Verification items for the finished model (mm, model axes). Coordinates: 2 decimals unless noted, no trailing zeros. Loops run counter-clockwise (first coordinate to the right, second up) from the corner with the lowest first, then second, coordinate; pieces in that order, holes last. Notation, with made-up numbers: (54.25, -23) - (81.25, -23) arc R8 cw to (81.25, -12) - close; hole circle Ø10 at (21, 78.5). An arc over 180 degrees is marked (long way). Answer as CSV lines item,"result". Start each with the question number.
1. Gauge pin test, flat ends, axial feed: P1, Ø12, axis at x = 40.5, y = -8, coming from the +Z side; P2, Ø1.5, axis at x = 68, z = 2.5, coming from the -Y side; P3, Ø1.5, axis at x = 51, z = 2, coming from the +Y side. Record the tip position at first contact, or that the pin passes through.
2. Cross-section at A-A (z = 1.9). State how many separate pieces and enclosed holes the cut face has, plus the area to 3 significant figures.
3. Material ranges on line 1 (Y direction, x = -18, z = 0.8); line 2 (Z direction, x = 44, y = 30.5); line 3 (Y direction, x = 68.5, z = 1.15), recorded low to high. Write a range as [from, to].
4. Cross-section at D-D (y = 29.5). Enter the section's corners in (x, z), plus the area to 3 significant figures.
5. Cross-section at B-B (x = 60.5). Enter the section's corners in (y, z), plus the area to 3 significant figures.
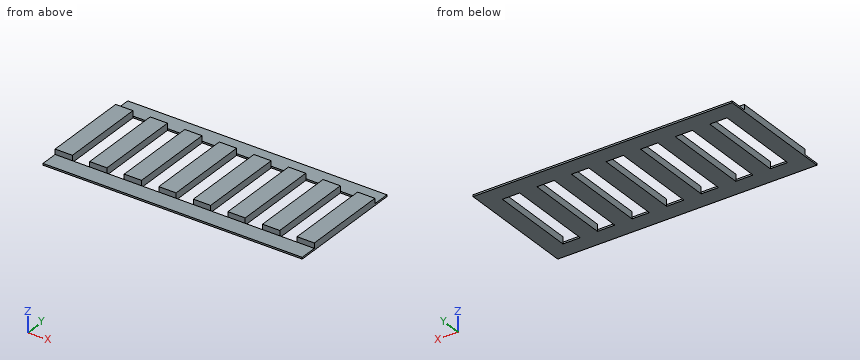
Autodesk Fusion 360 part; units mm, degrees
sketch "Sketch1" plane through (0, 0, 0) normal (0, 0, 1) x (1, 0, 0)
  line L0 (75, -35) -> (-75, -35)
  line L1 (-75, -35) -> (-75, 35)
  line L2 (-75, 35) -> (75, 35)
  line L3 (75, 35) -> (75, -35)
  line L4 (75, -35) -> (-75, 35) construction
  line L5 (-75, -35) -> (75, 35) construction
  line L6 (75, -25) -> (-75, -25)
  line L7 (-75, -25) -> (-75, 25)
  line L8 (-75, 25) -> (75, 25)
  line L9 (75, 25) -> (75, -25)
  line L10 (75, -25) -> (-75, 25) construction
  line L11 (-75, -25) -> (75, 25) construction
  line L12 (-75, 25) -> (-65, 25)
  line L13 (-65, 25) -> (-65, -25)
  line L14 (-65, -25) -> (-75, -25)
  line L15 (-75, -25) -> (-75, 25)
  line L16 (-55, 25) -> (-45, 25)
  line L17 (-45, 25) -> (-45, -25)
  line L18 (-45, -25) -> (-55, -25)
  line L19 (-55, -25) -> (-55, 25)
  line L20 (-35, 25) -> (-25, 25)
  line L21 (-25, 25) -> (-25, -25)
  line L22 (-25, -25) -> (-35, -25)
  line L23 (-35, -25) -> (-35, 25)
  line L24 (-15, 25) -> (-5, 25)
  line L25 (-5, 25) -> (-5, -25)
  line L26 (-5, -25) -> (-15, -25)
  line L27 (-15, -25) -> (-15, 25)
  line L28 (5, 25) -> (15, 25)
  line L29 (15, 25) -> (15, -25)
  line L30 (15, -25) -> (5, -25)
  line L31 (5, -25) -> (5, 25)
  line L32 (25, 25) -> (35, 25)
  line L33 (35, 25) -> (35, -25)
  line L34 (35, -25) -> (25, -25)
  line L35 (25, -25) -> (25, 25)
  line L36 (45, 25) -> (55, 25)
  line L37 (55, 25) -> (55, -25)
  line L38 (55, -25) -> (45, -25)
  line L39 (45, -25) -> (45, 25)
  line L40 (65, 25) -> (75, 25)
  line L41 (75, 25) -> (75, -25)
  line L42 (75, -25) -> (65, -25)
  line L43 (65, -25) -> (65, 25)
  dimension "d1" = 150
  dimension "d2" = 70
  dimension "d3" = 150
  dimension "d4" = 50
  dimension "d5" = 10
  dimension "d8" = 140
  dimension "d9" = 0
extrude "Extrude1" add sketch "Sketch1" along normal blind 4 contours L3 L6 L8 L9 L40 L41 L42 L43 | L1 L6 L7 L8 L12 L13 L14 L15 | L6 L8 L36 L37 L38 L39 | L6 L8 L16 L17 L18 L19 | L6 L8 L32 L33 L34 L35 | L6 L8 L20 L21 L22 L23 | L6 L8 L28 L29 L30 L31 | L6 L8 L24 L25 L26 L27 makes body 1 at (-31.6667, 8.3333, 0) makes body 2 at (-71.6667, 8.3333, 0) makes body 3 at (31.6667, -8.3333, 0) makes body 4 at (-51.6667, 8.3333, 0) makes body 5 at (68.3333, -8.3333, 0) makes body 6 at (11.6667, -8.3333, 0) makes body 7 at (51.6667, -8.3333, 0) makes body 8 at (-11.6667, 8.3333, 0)
extrude "Extrude2" add sketch "Sketch1" along normal blind 1 contours L0 L1 L3 L6 L14 L18 L22 L26 L30 L34 L38 L42 | L1 L2 L3 L8 L12 L16 L20 L24 L28 L32 L36 L40 bodies 1 2 3 4 5 6 7 8
Values follow:
1,P1,"stops at z = 4"
1,P2,"stops at y = -25"
1,P3,"stops at y = 25"
2,separate pieces,"8"
2,enclosed holes,"0"
2,area,"4,000 mm²"
3,line 1,"y = [-35, -25], [25, 35]"
3,line 2,"z = [0, 1]"
3,line 3,"y = [-25, 25]"
4,outline,"(-75, 0) - (75, 0) - (75, 1) - (-75, 1) - close"
4,area,"150 mm²"
5,outline,"(-35, 0) - (-25, 0) - (-25, 1) - (-35, 1) - close; (25, 0) - (35, 0) - (35, 1) - (25, 1) - close"
5,area,"20.0 mm²"
